Source: CAD feature listing. Evaluate the final solid. Frame: model axes, mm. A direction names the side the tool comes from. Round coordinates to 2 decimals unless told otherwise and drop trailing zeros. Write each loop counter-clockwise with the first axis right and the second up, starting at its lowest first coordinate (ties: lowest second). Pieces come first, ordered by that corner, then holes.
from build123d import *

# Parameters (mm, degrees)
BOSS_EXTRUDE3_DEPTH = 4
CUT_EXTRUDE3_REACH  = 6
SKETCH5_R           = 3
SKETCH5_R_2         = 7.5
SKETCH5_R_3         = 2.6


with BuildPart() as part:
    # Sketch1 → Boss-Extrude3 (new body)
    with BuildSketch(Plane(origin=(0, 0, 0), x_dir=(1, 0, 0), z_dir=(0, 1, 0))):
        Polygon((40.5, -35), (56.816666667, -90), (82, -90), (82, 90), (-82, 90), (-82, -90), (-56.816666667, -90), (-40.5, -35), align=None)
    extrude(amount=BOSS_EXTRUDE3_DEPTH)

    # Sketch5 → Cut-Extrude3 (cut, up to next)
    with BuildSketch(Plane(origin=(0, 4, 0), x_dir=(1, 0, 0), z_dir=(0, 1, 0)), mode=Mode.PRIVATE) as cut_extrude3_sk1:
        with Locations((62, -74.75)):
            Circle(SKETCH5_R)
    cut_extrude3_tool1 = extrude(cut_extrude3_sk1.sketch, amount=-CUT_EXTRUDE3_REACH, mode=Mode.PRIVATE) & part.part
    add(cut_extrude3_tool1.solids().sort_by_distance((62, 4, 74.75))[0], mode=Mode.SUBTRACT)
    # Sketch5 → Cut-Extrude3 (cut, up to next)
    with BuildSketch(Plane(origin=(0, 4, 0), x_dir=(1, 0, 0), z_dir=(0, 1, 0)), mode=Mode.PRIVATE) as cut_extrude3_sk2:
        with Locations((62, -19.99)):
            Circle(SKETCH5_R)
    cut_extrude3_tool2 = extrude(cut_extrude3_sk2.sketch, amount=-CUT_EXTRUDE3_REACH, mode=Mode.PRIVATE) & part.part
    add(cut_extrude3_tool2.solids().sort_by_distance((62, 4, 19.99))[0], mode=Mode.SUBTRACT)
    # Sketch5 → Cut-Extrude3 (cut, up to next)
    with BuildSketch(Plane(origin=(0, 4, 0), x_dir=(1, 0, 0), z_dir=(0, 1, 0)), mode=Mode.PRIVATE) as cut_extrude3_sk3:
        with Locations((-62, -74.75)):
            Circle(SKETCH5_R)
    cut_extrude3_tool3 = extrude(cut_extrude3_sk3.sketch, amount=-CUT_EXTRUDE3_REACH, mode=Mode.PRIVATE) & part.part
    add(cut_extrude3_tool3.solids().sort_by_distance((-62, 4, 74.75))[0], mode=Mode.SUBTRACT)
    # Sketch5 → Cut-Extrude3 (cut, up to next)
    with BuildSketch(Plane(origin=(0, 4, 0), x_dir=(1, 0, 0), z_dir=(0, 1, 0)), mode=Mode.PRIVATE) as cut_extrude3_sk4:
        with Locations((-62, -19.99)):
            Circle(SKETCH5_R)
    cut_extrude3_tool4 = extrude(cut_extrude3_sk4.sketch, amount=-CUT_EXTRUDE3_REACH, mode=Mode.PRIVATE) & part.part
    add(cut_extrude3_tool4.solids().sort_by_distance((-62, 4, 19.99))[0], mode=Mode.SUBTRACT)
    # Sketch5 → Cut-Extrude3 (cut, up to next)
    with BuildSketch(Plane(origin=(0, 4, 0), x_dir=(1, 0, 0), z_dir=(0, 1, 0)), mode=Mode.PRIVATE) as cut_extrude3_sk5:
        with Locations((0, -6.25)):
            Circle(SKETCH5_R_2)
    cut_extrude3_tool5 = extrude(cut_extrude3_sk5.sketch, amount=-CUT_EXTRUDE3_REACH, mode=Mode.PRIVATE) & part.part
    add(cut_extrude3_tool5.solids().sort_by_distance((0, 4, 6.25))[0], mode=Mode.SUBTRACT)
    # Sketch5 → Cut-Extrude3 (cut, up to next)
    with BuildSketch(Plane(origin=(0, 4, 0), x_dir=(1, 0, 0), z_dir=(0, 1, 0)), mode=Mode.PRIVATE) as cut_extrude3_sk6:
        with Locations((0, -22.5)):
            Circle(SKETCH5_R_3)
    cut_extrude3_tool6 = extrude(cut_extrude3_sk6.sketch, amount=-CUT_EXTRUDE3_REACH, mode=Mode.PRIVATE) & part.part
    add(cut_extrude3_tool6.solids().sort_by_distance((0, 4, 22.5))[0], mode=Mode.SUBTRACT)


solid = part.part
1) Section query C-C on z = 6.25. Return the cut outline in (x, y), then the cut area to 3 significant figures.
Taken from the geometry:
outline: (-82, 0) - (-7.5, 0) - (-7.5, 4) - (-82, 4) - close; (7.5, 0) - (82, 0) - (82, 4) - (7.5, 4) - close
area: 596 mm2
2) Reachability of faces 4 (the face through (59.619, 2.028, 21.815)), 5 (the face through (-1, 2, 35)) from +Z, -Z, +X, -X, +Y, -Y: full face, straight path, thin tool, end or side. Return the list, or none.
Taken from the geometry:
face 4: +Y, -Y
face 5: +Z, +Y, -Y
3) Contact query for flat-ended pins moving along their axis: P1, Ø7, axis at x = 0, z = 22.5, coming from the +Y side; P2, Ø1.2, axis at x = -12, y = 1.5, coming from the +Z side. Output: stop coordinate, or through.
Taken from the geometry:
P1: stops at y = 4
P2: stops at z = 35
4) Section query D-D on x = -62. Return the cut outline in (y, z), then the cut area to 3 significant figures.
Taken from the geometry:
outline: (0, -90) - (4, -90) - (4, 16.99) - (0, 16.99) - close; (0, 22.99) - (4, 22.99) - (4, 71.75) - (0, 71.75) - close; (0, 77.75) - (4, 77.75) - (4, 90) - (0, 90) - close
area: 672 mm2
5) Section query A-A on x = 0. Return the cut outline in (y, z).
Taken from the geometry:
outline: (0, -90) - (4, -90) - (4, -1.25) - (0, -1.25) - close; (0, 13.75) - (4, 13.75) - (4, 19.9) - (0, 19.9) - close; (0, 25.1) - (4, 25.1) - (4, 35) - (0, 35) - close
6) Section query B-B on y = 2.35. Return the cut outline in (x, z).
Taken from the geometry:
outline: (-82, -90) - (82, -90) - (82, 90) - (56.82, 90) - (40.5, 35) - (-40.5, 35) - (-56.82, 90) - (-82, 90) - close; hole circle Ø6 at (-62, 19.99); hole circle Ø6 at (-62, 74.75); hole circle Ø15 at (0, 6.25); hole circle Ø5.2 at (0, 22.5); hole circle Ø6 at (62, 19.99); hole circle Ø6 at (62, 74.75)
7) Material intervals for line 1 (Z direction, x = 0, y = 3.15); line 2 (Z direction, x = 62, y = 1.7); line 3 (X direction, y = 2.5, z = 74.75), sorted ascending.
Taken from the geometry:
line 1: z = -90 to -1.25, 13.75 to 19.9, 25.1 to 35
line 2: z = -90 to 16.99, 22.99 to 71.75, 77.75 to 90
line 3: x = -82 to -65, -59 to -52.29, 52.29 to 59, 65 to 82
8) Pull-direction query (Z, two-part tool) for faces 1 (the face through (82, 2, 1)), 2 (the face through (-0.976, 2.028, -1.186)), 3 (the face through (48.544, 1.972, 62.115)); classes: released by +Z, released by -Z, zero draft, split by the parting line, or undercut.
Taken from the geometry:
face 1: zero draft
face 2: undercut
face 3: released by +Z
